Source: CAD feature listing. Evaluate the final solid. Frame: model axes, mm. A direction names the side the tool comes from. Give positions to 0.01 mm unless a question says otherwise; leave off trailing zeros. Write each loop counter-clockwise with the first axis right and the second up, starting at its lowest first coordinate (ties: lowest second). Pieces come first, ordered by that corner, then holes. Notation, with made-up numbers: (55.25, -32) -> (74.25, -32) arc R13 cw to (74.25, -27) -> close; hole circle Ø6 at (-1.75, 61.5). An arc over 180 degrees is marked (long way). Write item = value, one per line.
from build123d import *

# Parameters (mm, degrees)
F2_R     = 2.6
F3_DEPTH = 25
F4_R     = 4
F5_DEPTH = 25


with BuildPart() as f1:
    # F0 (on Front) → F1 (revolve)
    with BuildSketch(Plane.XZ):
        Polygon((-18.202801, -2.841857), (8.197199, -2.841857), (8.197199, 7.658143), (-12.202801, 7.658143), (-12.202801, 17.558143), (-18.202801, 17.558143), align=None)
    revolve(axis=Axis((2.917131, 0, -10.841857), (1, 0, 0)))

    # F2 (on face) → F3 (cut)
    with BuildSketch(Plane(origin=(-18.202801, 0, 0), x_dir=(0, -1, 0), z_dir=(-1, 0, 0))):
        with Locations((0, 12.908143)):
            Circle(F2_R)
        with Locations((-20.568103, 1.033143)):
            Circle(F2_R)
        with Locations((-20.568103, -22.716857)):
            Circle(F2_R)
        with Locations((0, -34.591857)):
            Circle(F2_R)
        with Locations((20.568103, -22.716857)):
            Circle(F2_R)
        with Locations((20.568103, 1.033143)):
            Circle(F2_R)
    extrude(amount=-F3_DEPTH, mode=Mode.SUBTRACT)

    # F4 (on Front) → F5 (cut)
    with BuildSketch(Plane.XZ):
        with Locations((-2.002801, -10.072675)):
            Circle(F4_R)
    extrude(amount=-F5_DEPTH, mode=Mode.SUBTRACT)


solid = f1.part
1) Contact query for flat-ended pins moving along their axis: pin 1 (6 mm diameter, centred on y = 20.57, z = 1.03, fed in from +X); pin 2 (3 mm diameter, centred on x = -14, z = -11.5, fed in from -Y); pin 3 (3 mm diameter, centred on x = -4.5, z = -16.5, fed in from +Y). Output: stop coordinate, or through.
Computed:
pin_1 = -12.2
pin_2 = -28.4
pin_3 = 18.03
2) Draft query along Y for faces 1 (the flat face through (-12.203, 19, -10)), 2 (the cylindrical face through (-4.818, -7.932, -11.883)), 3 (the cylindrical face through (-15.245, -1.249, -39.214)). Return one class per face: pulls with the +Y half, pulls with the -Y half, needs draft (parallel to the pull), parting line crosses it, or undercut.
Computed:
face_1 = needs draft
face_2 = undercut
face_3 = parting line crosses it
3) Cut plane A-A (y = 0). Return the cut outline in (x, z).
Computed:
outline = (-18.2, -39.24) -> (-12.2, -39.24) -> (-12.2, -37.19) -> (-18.2, -37.19) -> close; (-18.2, -31.99) -> (-12.2, -31.99) -> (-12.2, -29.34) -> (8.2, -29.34) -> (8.2, -18.84) -> (-18.2, -18.84) -> close; (-18.2, -2.84) -> (8.2, -2.84) -> (8.2, 7.66) -> (-12.2, 7.66) -> (-12.2, 10.31) -> (-18.2, 10.31) -> close; (-18.2, 15.51) -> (-12.2, 15.51) -> (-12.2, 17.56) -> (-18.2, 17.56) -> close
4) Cut plane D-D (x = 6). Return the cut outline in (y, z).
Computed:
outline = circle Ø37 at (0, -10.84); hole circle Ø16 at (0, -10.84)
5) Cut plane C-C (y = -20). Return the cut outline in (x, z).
Computed:
outline = (-18.2, -31.01) -> (-12.2, -31.01) -> (-12.2, -25.25) -> (-18.2, -25.25) -> close; (-18.2, -20.18) -> (-12.2, -20.18) -> (-12.2, -1.5) -> (-18.2, -1.5) -> close; (-18.2, 3.57) -> (-12.2, 3.57) -> (-12.2, 9.32) -> (-18.2, 9.32) -> close
6) Material intervals for L1, parallel to Z at x = -14, y = 0; L2, parallel to X at y = 18, z = 2; L3, parallel to Z at x = -12, y = 0.5, sorted ascending.
Computed:
L1 = -39.24 to -37.19, -31.99 to -18.84, -2.84 to 10.31, 15.51 to 17.56
L2 = -18.2 to -12.2
L3 = -29.34 to -18.83, -2.86 to 7.65
7) Access query for faces 4 (the cylindrical face through (0.15, 12.38, -6.7)), 5 (the cylindrical face through (-2.146, 16.413, -2.305)), 6 (the flat face through (-18.203, 6, -5)). Directions: +Z, -Z, +X, -X, +Y, -Y. A direction counts if a zero-diameter tool reaches every point of the face in a straight line with its end or side. Return the directions, or none.
Computed:
face_4 = +Y
face_5 = +X
face_6 = +Z, -Z, -X, +Y, -Y
8) Cut plane B-B (z = -33.5). Return the cut outline in (x, y).
Computed:
outline = (-18.2, -17.12) -> (-12.2, -17.12) -> (-12.2, -2.36) -> (-18.2, -2.36) -> close; (-18.2, 2.36) -> (-12.2, 2.36) -> (-12.2, 17.12) -> (-18.2, 17.12) -> close
